Verification items for the finished model (mm, model axes). A direction names the side the tool comes from. Round coordinates to 2 decimals unless told otherwise and drop trailing zeros. Order: outer loops, then holes, each group sorted by start corner. A loop starts at its lowest first (then second) coordinate and runs counter-clockwise, first axis right, second up. Notation, with made-up numbers: (24.25, 76) -> (43.25, 76) arc R29 ccw to (43.25, 115) -> close; hole circle Ø7 at (-23.75, 73.25). An arc over 180 degrees is marked (long way). Put each result on its own line as item: value.
```python
from build123d import *

# Parameters (mm, degrees)
FILLET1_R   = 0.2
HEX_2_DEPTH = 1.3


with BuildPart() as part:
    # BodySke → BaseBody (revolve)
    with BuildSketch(Plane.XY):
        with BuildLine():
            Line((22.2, 0), (22.2, 1.61))
            Line((22.2, 1.61), (21.81, 2))
            Line((21.81, 2), (2.2, 2))
            Line((2.2, 2), (2.2, 3.8))
            Line((2.2, 3.8), (1.82, 3.8))
            ThreePointArc((1.82, 3.8), (0.762013659, 2.991755338), (0, 1.9))
            Line((0, 1.9), (0, 0))
            Line((0, 0), (22.2, 0))
        make_face()
    revolve(axis=Axis((0, 0, 0), (1, 0, 0)))

    # Fillet1
    fillet1_edges = [part.edges().sort_by_distance(p)[0] for p in [
        (2.2, -2, 0),
    ]]
    fillet(fillet1_edges, radius=FILLET1_R)

    # Sketch2 → PreBroach (revolve, cut)
    with BuildSketch(Plane.XY):
        Polygon((0, 1.25), (1.3, 1.25), (2.021687836, 0), (0, 0), align=None)
    revolve(axis=Axis((0, 0, 0), (1, 0, 0)), mode=Mode.SUBTRACT)

    # Sketch3 → Hex 2 (cut)
    with BuildSketch(Plane(origin=(0, 0, 0), x_dir=(0, 0, -1), z_dir=(1, 0, 0))):
        Polygon((-1.25, -0.721687836), (-1.25, 0.721687836), (0, 1.443375673), (1.25, 0.721687836), (1.25, -0.721687836), (0, -1.443375673), align=None)
    extrude(amount=HEX_2_DEPTH, mode=Mode.SUBTRACT)


solid = part.part
```
Item 1: Tool access check on faces 1 (the face through (0.641, 1.088, -0.616)), 2 (the face through (22.2, 0, 0)). Record the directions out of +Z, -Z, +X, -X, +Y, -Y that give a thin tool (end or side, any length) a straight path to the whole face; none if there is none.
Geometry check:
face 1: -X
face 2: +Z, -Z, +X, +Y, -Y
Item 2: Sectioned sample at C-C, the plane y = -2.75. Record the boundary of the cut face in (x, z).
Geometry check:
outline: (1.82, -2.62) -> (2.2, -2.62) -> (2.2, 2.62) -> (1.82, 2.62) arc R3.34 ccw to start
Item 3: Material ranges on line 1 along Z through (x, y) = (14.75, 0); line 2 along X through (y, z) = (1.75, -3.25); line 3 along X through (y, z) = (-0.25, 2.75), recorded low to high.
Geometry check:
line 1: -2 to 2
line 2: 1.63 to 2.2
line 3: 0.56 to 2.2
Item 4: Sectioned sample at B-B, the plane z = -2.5. Record the boundary of the cut face in (x, y), then the cut area to 3 significant figures.
Geometry check:
outline: (1.82, -2.86) -> (2.2, -2.86) -> (2.2, 2.86) -> (1.82, 2.86) arc R3.53 ccw to start
area: 8.04 mm2
Item 5: Sectioned sample at A-A, the plane x = 18. Record the boundary of the cut face in (y, z), then the cut area to 3 significant figures.
Geometry check:
outline: circle Ø4 at (0, 0)
area: 12.6 mm2
Item 6: Release check for a two-part mould opening along Y. For faces 3 (the face through (12, 0, -2)), 4 (the face through (0.64, 1.08, 0.63)), 5 (the face through (2.2, -2, -2)) record: pulls with the +Y half, pulls with the -Y half, needs draft (parallel to the pull), parting line crosses it, or undercut.
Geometry check:
face 3: parting line crosses it
face 4: undercut
face 5: needs draft
Item 7: Depth check by flat-ended pin: pin 1 Ø1.4 at (x, y) = (0.5, 0) entering from -Z; pin 2 Ø2.5 at (y, z) = (1.5, 1.5) entering from +X; pin 3 Ø4 at (x, y) = (11, -0.5) entering from +Z; pin 4 Ø0.6 at (x, y) = (0.5, -0.5) entering from +Z. Enter the tip coordinate at first touch or a pass-through.
Geometry check:
pin 1: z = -3.39
pin 2: x = 22.2
pin 3: z = 2
pin 4: z = 2.99
